```python
from build123d import *

# Parameters (mm, degrees)
F0_W     = 31.838607043
F0_H     = 24.8093027622
F1_DEPTH = 25.4
F2_R     = 6.6170085052
F3_DEPTH = 40.64
F4_DEPTH = 17.272
F5_R     = 14.8582779771
F5_R_2   = 10.1809706262
F6_DEPTH = 51.816


with BuildPart() as f1:
    # F0 (on Top) → F1 (new body)
    with BuildSketch(Plane.XY):
        Rectangle(F0_W, F0_H)
    extrude(amount=F1_DEPTH)

    # F2 (on Right) → F3 (join, symmetric)
    with BuildSketch(Plane.YZ):
        with Locations((0.0505595074, 14.8865826207)):
            Circle(F2_R)
    extrude(amount=F3_DEPTH, both=True)

    # F4 (add, symmetric): faces of the model
    f4_faces = [f1.faces().sort_by_distance(p)[0] for p in [
        (-40.64, 0.0505595074, 14.8865826207),
        (40.64, 0.0505595074, 14.8865826207),
    ]]
    extrude(f4_faces, amount=F4_DEPTH, both=True, dir=(-1, 0, 0))

    # F5 (on Right) → F6 (join, symmetric)
    with BuildSketch(Plane.YZ):
        with Locations((0, 10.337209329)):
            Circle(F5_R)
        with Locations((0, 10.337209329)):
            Circle(F5_R_2, mode=Mode.SUBTRACT)
    extrude(amount=F6_DEPTH, both=True)


solid = f1.part
```
The model under review builds one solid part; all positions refer to its coordinate system, in mm. A direction names the side the tool comes from. Round coordinates to 2 decimals unless told otherwise and drop trailing zeros. Loops run counter-clockwise (first coordinate to the right, second up) from the corner with the lowest first, then second, coordinate; pieces in that order, holes last.
Item 1: For line 1 (Z direction, x = -26, y = 0); line 2 (Y direction, x = -17.5, z = 11); line 3 (Y direction, x = -33.5, z = 9.5), list the stretches that pass through material, from the lowest coordinate up.
Determined:
line 1: z = -4.52 to 0.16, 8.27 to 25.2
line 2: y = -14.84 to -10.16, -5.3 to 5.41, 10.16 to 14.84
line 3: y = -14.83 to -10.15, -3.79 to 3.89, 10.15 to 14.83
Item 2: For faces 1 (the face through (0.725, 6.856, -2.845)), 2 (the face through (-15.919, 0, 7)), 3 (the face through (51.816, -3.5, 0.6)), list the 3-axis set-ups (+Z, -Z, +X, -X, +Y, -Y) from which the entire face can be reached by the end or side of a thin tool; tool diameter is ignored.
Determined:
face 1: none
face 2: -X
face 3: +X
Item 3: Take a section at A-A (x = -7). Write out the cut boundary in (y, z), then the cut area to 3 significant figures.
Determined:
outline: (-12.4, 0) - (-10.67, 0) arc R14.86 ccw to (10.67, 0) - (12.4, 0) - (12.4, 2.16) arc R14.86 ccw to (12.4, 18.52) - (12.4, 25.4) - (-12.4, 25.4) - (-12.4, 18.52) arc R14.86 ccw to (-12.4, 2.16) - close
area: 751 mm2
Item 4: Clearance check with flat-ended pins moving along their axes: pin 1 Ø0.9 at (y, z) = (11.5, 1) entering from +X; pin 2 Ø6 at (x, y) = (-33.5, -9) entering from -Z; pin 3 Ø6 at (x, y) = (9.5, -0.5) entering from -Z; pin 4 Ø5 at (x, y) = (35, 5) entering from +Z. State where each tip first meets the part, or that it passes through.
Determined:
pin 1: stops at x = 51.82
pin 2: stops at z = -3.26
pin 3: stops at z = -4.52
pin 4: stops at z = 24.98
Item 5: Take a section at B-B (y = 0.5). Write out the cut boundary in (x, z), then the cut area to 3 significant figures.
Determined:
outline: (-57.91, 8.28) - (-15.92, 8.28) - (-15.92, 0.17) - (-51.82, 0.17) - (-51.82, -4.51) - (51.82, -4.51) - (51.82, 0.17) - (15.92, 0.17) - (15.92, 8.28) - (57.91, 8.28) - (57.91, 21.49) - (51.82, 21.49) - (51.82, 25.19) - (15.92, 25.19) - (15.92, 25.4) - (-15.92, 25.4) - (-15.92, 25.19) - (-51.82, 25.19) - (-51.82, 21.49) - (-57.91, 21.49) - close
area: 2,660 mm2
Item 6: Take a section at D-D (x = -50). Write out the cut boundary in (y, z).
Determined:
outline: circle Ø29.72 at (0, 10.34); hole (-4.93, 19.25) arc R10.18 ccw (long way) to (5.12, 19.13) arc R6.62 cw (long way) to start
Item 7: Mouldability with a two-part tool opening along Z and no side actions: class faces 4 (the face through (-34.12, -0.49, 0.17)), 5 (the face through (0, -12.405, 1)), 6 (the face through (0, 0, 25.4)) as released by +Z, released by -Z, zero draft, split by the parting line, or undercut.
Determined:
face 4: undercut
face 5: zero draft
face 6: released by +Z
Item 8: Take a section at C-C (z = 20.5). Write out the cut boundary in (x, y), then the cut area to 3 significant figures.
Determined:
outline: (-57.91, -3.45) - (-51.82, -3.45) - (-51.82, -10.84) - (-15.92, -10.84) - (-15.92, -12.4) - (15.92, -12.4) - (15.92, -10.84) - (51.82, -10.84) - (51.82, -3.45) - (57.91, -3.45) - (57.91, 3.55) - (51.82, 3.55) - (51.82, 10.84) - (15.92, 10.84) - (15.92, 12.4) - (-15.92, 12.4) - (-15.92, 10.84) - (-51.82, 10.84) - (-51.82, 3.55) - (-57.91, 3.55) - close
area: 2,430 mm2
